For this review, take the finished solid that the model builds, in its own axes (mm). Face numbers are marked on the shaded views. A direction names the side the tool comes from. Coordinates: 2 decimals unless noted, no trailing zeros. Write each loop counter-clockwise with the first axis right and the second up, starting at its lowest first coordinate (ties: lowest second). Pieces come first, ordered by that corner, then holes.
1) We need section B-B on z = 5.5. Give the number of separate pieces and of enclosed holes in the cut face, then the cut area to 3 significant figures.
2) Mouldability with a two-part tool opening along Y and no side actions: class the marked faces 4, 5 and 6 as pulls with the +Y half, pulls with the -Y half, needs draft (parallel to the pull), parting line crosses it, or undercut.
3) We need section A-A on x = 4.5. Write out the cut boundary in (y, z).
4) To check wall thickness, follow line 1 along X through (y, z) = (8.5, 6.25) (3 decimals); line 2 along Y through (x, z) = (11.5, 8); line 3 along Z through (x, y) = (32, 2). State the ranges of each line that lie inside material, in increasing order.
5) For the marked faces 1, 2 and 3, list the 3-axis set-ups (+Z, -Z, +X, -X, +Y, -Y) from which the entire face can be reached by the end or side of a thin tool; tool diameter is ignored.
6) We need section D-D on y = 22. Write out the cut boundary in (x, z).
7) Insertion check: P1, Ø3.5, axis at x = 33, z = 7, coming from the +Y side; P2, Ø6, axis at y = 39, z = 7.5, coming from the +X side; P3, Ø3, axis at y = 10, z = 5.5, coming from the +X side. Each pin has a flat end and moves straight along its axis. Give the tip position at first contact, or say it passes through.
8) We need section C-C on y = 14.5. Write out the cut boundary in (x, z), then the cut area to 3 significant figures.
from build123d import *

# Parameters (mm, degrees)
EXTRUDE_1_DEPTH     = 11
SKETCH_2_R          = 2.15
CUT_EXTRUDE_1_DEPTH = 69.767724988
CUT_EXTRUDE_2_DEPTH = 4
FILLET_1_R          = 2
CHAMFER_1_SIZE      = 4
FILLET_2_R          = 2
FILLET_3_R          = 0.5
SKETCH_4_R          = 2.1
CUT_EXTRUDE_3_DEPTH = 69.767724988


with BuildPart() as part:
    # 草图1 → 凸台-拉伸1 (new body)
    with BuildSketch(Plane.XY):
        Polygon((0, 16), (16, 0), (48, 0), (48, 12), (24, 12), (12, 24), (12, 48), (0, 48), align=None)
    extrude(amount=EXTRUDE_1_DEPTH)

    # 草图2 → 切除-拉伸1 (cut, symmetric)
    with BuildSketch(Plane.ZY):
        with Locations(Location((5.5, 40, 0), (0, 0, 270))):
            Circle(SKETCH_2_R)
        with Locations(Location((5.5, 32, 0), (0, 0, 270))):
            Circle(SKETCH_2_R)
    cut_extrude_1 = extrude(amount=CUT_EXTRUDE_1_DEPTH, both=True, mode=Mode.SUBTRACT)

    # 草图3 → 切除-拉伸2 (cut)
    with BuildSketch(Plane(origin=(12, 0, 0), x_dir=(0, 0, -1), z_dir=(1, 0, 0))):
        Polygon((-1.314210548, 40), (-3.407105274, 43.625), (-7.592894726, 43.625), (-9.685789452, 40), (-7.592894726, 36.375), (-3.407105274, 36.375), align=None)
        Polygon((-1.314210548, 32), (-3.407105274, 35.625), (-7.592894726, 35.625), (-9.685789452, 32), (-7.592894726, 28.375), (-3.407105274, 28.375), align=None)
    cut_extrude_2 = extrude(amount=-CUT_EXTRUDE_2_DEPTH, mode=Mode.SUBTRACT)

    # 镜向1: 切除-拉伸1, 切除-拉伸2 across plane
    add(cut_extrude_1.mirror(Plane(origin=(0, 0, 0), x_dir=(0, 0, 1), z_dir=(-0.7071067811865475, 0.7071067811865476, 0))), mode=Mode.SUBTRACT)
    add(cut_extrude_2.mirror(Plane(origin=(0, 0, 0), x_dir=(0, 0, 1), z_dir=(-0.7071067811865475, 0.7071067811865476, 0))), mode=Mode.SUBTRACT)

    # 圆角1
    fillet_1_edges = [part.edges().sort_by_distance(p)[0] for p in [
        (12, 24, 5.5),
        (24, 12, 5.5),
        (16, 0, 5.5),
        (0, 16, 5.5),
    ]]
    fillet(fillet_1_edges, radius=FILLET_1_R)

    # 倒角1
    chamfer_1_edges = [part.edges().sort_by_distance(p)[0] for p in [
        (12, 48, 5.5),
        (48, 12, 5.5),
    ]]
    chamfer(chamfer_1_edges, length=CHAMFER_1_SIZE)

    # 圆角2
    fillet_2_edges = [part.edges().sort_by_distance(p)[0] for p in [
        (48, 4, 0),
        (4, 48, 0),
        (10, 46, 0),
        (46, 10, 0),
        (4, 48, 11),
        (10, 46, 11),
        (46, 10, 11),
        (48, 4, 11),
    ]]
    fillet(fillet_2_edges, radius=FILLET_2_R)

    # 圆角3
    fillet_3_edges = [part.edges().sort_by_distance(p)[0] for p in [
        (28.375, 10, 3.407105274),
        (32, 10, 1.314210548),
        (35.625, 10, 3.407105274),
        (35.625, 10, 7.592894726),
        (32, 10, 9.685789452),
        (28.375, 10, 7.592894726),
        (10, 40, 1.314210548),
        (10, 36.375, 3.407105274),
        (10, 36.375, 7.592894726),
        (10, 40, 9.685789452),
        (10, 43.625, 7.592894726),
        (10, 43.625, 3.407105274),
        (10, 32, 1.314210548),
        (10, 28.375, 3.407105274),
        (10, 28.375, 7.592894726),
        (10, 32, 9.685789452),
        (10, 35.625, 7.592894726),
        (10, 35.625, 3.407105274),
        (36.375, 10, 3.407105274),
        (40, 10, 1.314210548),
        (43.625, 10, 3.407105274),
        (43.625, 10, 7.592894726),
        (40, 10, 9.685789452),
        (36.375, 10, 7.592894726),
    ]]
    fillet(fillet_3_edges, radius=FILLET_3_R)

    # 草图4 → 切除-拉伸3 (cut, through all)
    with BuildSketch(Plane.XY.offset(11)):
        with Locations((13, 13)):
            Circle(SKETCH_4_R)
    extrude(amount=-CUT_EXTRUDE_3_DEPTH, mode=Mode.SUBTRACT)


solid = part.part
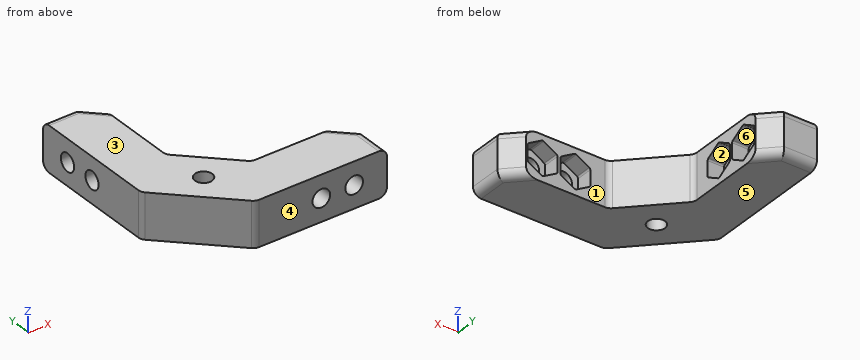
Result:
1. separate pieces: 5
1. enclosed holes: 1
1. area: 669 mm2
2. face 4: pulls with the -Y half
2. face 5: needs draft
2. face 6: undercut
3. outline: (11.5, 0) - (46, 0) arc R2 ccw to (48, 2) - (48, 9) arc R2 ccw to (46, 11) - (11.5, 11) - close; hole circle Ø4.3 at (32, 5.5); hole circle Ø4.3 at (40, 5.5)
4. line 1: x = 7.5 to 28.375, 35.625 to 36.375, 43.625 to 47.5
4. line 2: y = 4.5 to 11.53, 14.47 to 29.08, 34.92 to 37.08, 42.92 to 44.5
4. line 3: z = 0 to 3.35, 7.65 to 11
5. face 1: +Z, -Z, +X, +Y
5. face 2: +X
5. face 3: +Z, +X, -X, +Y, -Y
6. outline: (0, 0) - (14, 0) - (14, 11) - (0, 11) - close
7. P1: stops at y = 8
7. P2: stops at x = 12
7. P3: stops at x = 47.5
8. outline: (1.5, 0) - (11.53, 0) - (11.53, 11) - (1.5, 11) - close; (14.47, 0) - (21.5, 0) - (21.5, 11) - (14.47, 11) - close
8. area: 188 mm2
